```python
from build123d import *

# Parameters (mm, degrees)
F0_W     = 50
F0_H     = 40
F1_DEPTH = 10
F3_DEPTH = 40
F5_W     = 44
F5_H     = 10
F6_DEPTH = 18
F7_R     = 4.99999


# Not quite as in the source:
# - a fillet or chamfer is up to 0.001 mm smaller than in the source, because OpenCascade refuses the exact size


with BuildPart() as f1:
    # F0 (on Top) → F1 (new body)
    with BuildSketch(Plane.XY):
        Rectangle(F0_W, F0_H)
    extrude(amount=F1_DEPTH)

    # F2 (on face) → F3 (cut)
    with BuildSketch(Plane.XZ.offset(20)):
        with BuildLine():
            Line((-25, 10), (-25, 9.6663655309))
            ThreePointArc((-25, 9.6663655309), (0.0065046461, 7.0000153387), (25, 9.7856728837))
            Line((25, 9.7856728837), (25, 10))
            Line((25, 10), (-25, 10))
        make_face()
    extrude(amount=-F3_DEPTH, mode=Mode.SUBTRACT)

    # F5 (on offset) → F6 (cut)
    with BuildSketch(Plane.XY.offset(10)):
        with Locations((0, 12)):
            Rectangle(F5_W, F5_H)
        with Locations((0, -12)):
            Rectangle(F5_W, F5_H)
    extrude(amount=-F6_DEPTH, mode=Mode.SUBTRACT)

    # F7 (radius 5 in the source; OpenCascade refuses exactly that, so slightly less here)
    f7_edges = [f1.edges().sort_by_distance(p)[0] for p in [
        (-22, 17, 4.52656),
        (22, 17, 4.578769),
        (-22, -7, 4.52656),
        (22, -7, 4.578769),
        (-22, -17, 4.52656),
        (22, -17, 4.578769),
        (22, 7, 4.578769),
        (-22, 7, 4.52656),
    ]]
    fillet(f7_edges, radius=F7_R)


solid = f1.part
```
The listing builds one solid part. Answer for the finished solid, in the listing's coordinates (mm). A direction names the side the tool comes from. Give positions to 0.01 mm unless a question says otherwise; leave off trailing zeros. Order: outer loops, then holes, each group sorted by start corner. A loop starts at its lowest first (then second) coordinate and runs counter-clockwise, first axis right, second up. Notation, with made-up numbers: (8, 52) -> (15, 52) arc R22 cw to (15, 89) -> close; hole circle Ø8 at (-28.5, 77). An arc over 180 degrees is marked (long way). One line per item, written item: value.
1) Find section A-A, the plane z = 1. Count the separate pieces of the cut face and the enclosed holes in it, plus the area to 3 significant figures.
Reported:
separate pieces: 1
enclosed holes: 2
area: 1,160 mm^2
2) Find section C-C, the plane y = -15. Determine the outline of the cut face in (x, z).
Reported:
outline: (-25, 0) -> (-21, 0) -> (-21, 8.87) arc R116 cw to (-25, 9.67) -> close; (21, 0) -> (25, 0) -> (25, 9.79) arc R116 cw to (21, 8.97) -> close
3) Find section B-B, the plane x = 12. Determine the outline of the cut face in (y, z).
Reported:
outline: (-20, 0) -> (-17, 0) -> (-17, 7.65) -> (-20, 7.65) -> close; (-7, 0) -> (7, 0) -> (7, 7.65) -> (-7, 7.65) -> close; (17, 0) -> (20, 0) -> (20, 7.65) -> (17, 7.65) -> close
4) Find section D-D, the plane x = 18. Determine the outline of the cut face in (y, z).
Reported:
outline: (-20, 0) -> (-16.9, 0) -> (-16.9, 8.45) -> (-20, 8.45) -> close; (-7.1, 0) -> (7.1, 0) -> (7.1, 8.45) -> (-7.1, 8.45) -> close; (16.9, 0) -> (20, 0) -> (20, 8.45) -> (16.9, 8.45) -> close
5) Determine the mould class of faces 1 (the cylindrical face through (20, -16, 5)), 2 (the flat face through (25, 0, 5)), 3 (the flat face through (-25, 0, 5)) for opening direction X: pulls with the +X half, pulls with the -X half, needs draft (parallel to the pull), parting line crosses it, or undercut.
Reported:
face 1: undercut
face 2: pulls with the +X half
face 3: pulls with the -X half
6) A tool of negligible diameter and unlimited length cuts with its end or side. For faces 4 (the flat face through (0, -7, 4)), 5 (the flat face through (0, -20, 4)), from which of +Z, -Z, +X, -X, +Y, -Y can it reach the whole face along a straight path? Write none if from no direction.
Reported:
face 4: +Z, -Z
face 5: +Z, -Z, +X, -X, -Y
7) Find the intervals of material crossed by line 1 (Y direction, x = 9, z = 0.5); line 2 (X direction, y = -16, z = 0.75); line 3 (Y direction, x = -21.5, z = 6.75), in increasing order.
Reported:
line 1: y = -20 to -17, -7 to 7, 17 to 20
line 2: x = -25 to -20, 20 to 25
line 3: y = -20 to -14.18, -9.82 to 9.82, 14.18 to 20
